The listing builds one solid part. Answer for the finished solid, in the listing's coordinates (mm). Face numbers are marked on the shaded views. A direction names the side the tool comes from. Round coordinates to 2 decimals unless told otherwise and drop trailing zeros. Loops run counter-clockwise (first coordinate to the right, second up) from the corner with the lowest first, then second, coordinate; pieces in that order, holes last. Notation, with made-up numbers: (85, 10) - (107, 10) arc R10 ccw to (107, 18) - close; hole circle Ø11 at (70, -2). An arc over 180 degrees is marked (long way). Write item = value, one per line. Start each with the question number.
1) Section B-B, the plane y = -5.3 is taken. Determine the outline of the cut face in (x, z), and give its area (3 significant figures).
2) Section C-C, the plane x = -13 is taken. Determine the outline of the cut face in (y, z).
3) Given pin 1 Ø13 at (x, z) = (5.5, 10.5) entering from +Y; pin 2 Ø3 at (x, z) = (13, 13) entering from +Y; pin 3 Ø8 at (x, z) = (-11, -11.5) entering from +Y, each flat-ended and moving along its own axis, determine where each tip first touches the part or whether it passes through.
4) Section D-D, the plane x = -4 is taken. Determine the outline of the cut face in (y, z).
5) Straight lines are drawn through the part: line 1 along Z through (x, y) = (-13, -4.3); line 2 along Z through (x, y) = (-7.5, -4.75). For each, find the intervals that lie inside material, in ascending order.
6) A tool of negligible diameter and unlimited length cuts with its end or side. For the marked faces 1, 2, 3 and 4, from which of +Z, -Z, +X, -X, +Y, -Y can it reach the whole face along a straight path? Write none if from no direction.
7) Section A-A, the plane z = 13 is taken. Determine the outline of the cut face in (x, y).
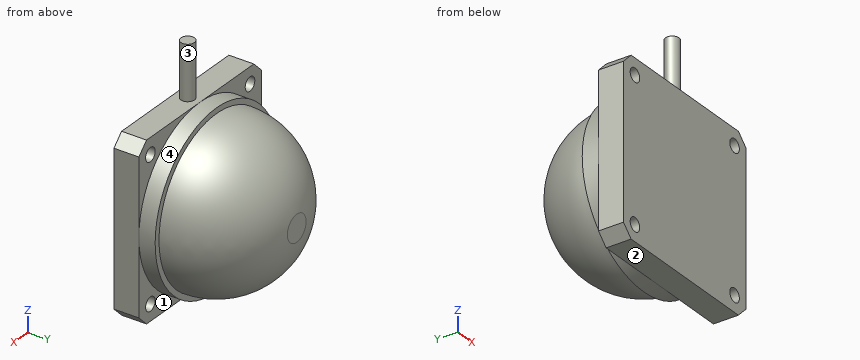
from build123d import *

# Parameters (mm, degrees)
SKETCH2_R             = 16
BOSS_EXTRUDE1_DEPTH   = 3
SKETCH3_W             = 32
SKETCH3_H             = 32
BOSS_EXTRUDE2_DEPTH   = 4.6
F_2_5MM_DOWEL_HOLE1_D = 2.5
CHAMFER1_SIZE         = 2
SKETCH11_R            = 1.25
BOSS_EXTRUDE3_DEPTH   = 10
SKETCH12_R            = 16
CUT_EXTRUDE1_DEPTH    = 38.865023439


with BuildPart() as part:
    # Sketch1 → Revolve1 (revolve)
    with BuildSketch(Plane.XY):
        with BuildLine():
            Line((0, 0), (15, 0))
            ThreePointArc((15, 0), (10.606601718, 10.606601718), (0, 15))
            Line((0, 15), (0, 0))
        make_face()
    revolve(axis=Axis((0, 15, 0), (0, -1, 0)))

    # Sketch2 → Boss-Extrude1 (add)
    with BuildSketch(Plane.XZ):
        Circle(SKETCH2_R)
    extrude(amount=BOSS_EXTRUDE1_DEPTH)

    # Sketch3 → Boss-Extrude2 (add)
    with BuildSketch(Plane.XZ.offset(3)):
        Rectangle(SKETCH3_W, SKETCH3_H)
    extrude(amount=BOSS_EXTRUDE2_DEPTH)

    # Ø2.5mm Dowel Hole1 (through all)
    with Locations(Plane(origin=(0, -3, 0), x_dir=(1, 0, 0), z_dir=(0, 1, 0))):
        with Locations((-13, 13), (13, -13), (13, 13), (-13, -13)):
            Hole(F_2_5MM_DOWEL_HOLE1_D / 2)

    # Chamfer1
    chamfer1_edges = [part.edges().sort_by_distance(p)[0] for p in [
        (16, -5.3, -16),
        (16, -5.3, 16),
        (-16, -5.3, 16),
        (-16, -5.3, -16),
    ]]
    chamfer(chamfer1_edges, length=CHAMFER1_SIZE)

    # Sketch11 → Boss-Extrude3 (add)
    with BuildSketch(Plane.XY.offset(16)):
        with Locations(Location((0, -5.3, 0), (0, 0, 180))):
            Circle(SKETCH11_R)
    extrude(amount=BOSS_EXTRUDE3_DEPTH)

    # Sketch12 → Cut-Extrude1 (cut, through all)
    with BuildSketch(Plane(origin=(0, 14.8, 0), x_dir=(1, 0, 0), z_dir=(0, 1, 0))):
        Circle(SKETCH12_R)
    extrude(amount=CUT_EXTRUDE1_DEPTH, mode=Mode.SUBTRACT)


solid = part.part
Geometry check:
q1.outline = (-16, -14) - (-14, -16) - (14, -16) - (16, -14) - (16, 14) - (14, 16) - (1.25, 16) - (1.25, 26) - (-1.25, 26) - (-1.25, 16) - (-14, 16) - (-16, 14) - close; hole circle Ø2.5 at (-13, -13); hole circle Ø2.5 at (-13, 13); hole circle Ø2.5 at (13, -13); hole circle Ø2.5 at (13, 13)
q1.area = 1,020 mm2
q2.outline = (-7.6, -16) - (-3, -16) - (-3, -14.25) - (-7.6, -14.25) - close; (-7.6, -11.75) - (-3, -11.75) - (-3, -9.33) - (0, -9.33) - (0, -7.48) arc R7.48 ccw to (0, 7.48) - (0, 9.33) - (-3, 9.33) - (-3, 11.75) - (-7.6, 11.75) - close; (-7.6, 14.25) - (-3, 14.25) - (-3, 16) - (-7.6, 16) - close
q3.pin_1 = 14.01
q3.pin_2 = -3
q3.pin_3 = 9.11
q4.outline = (-7.6, -16) - (-3, -16) - (-3, -15.49) - (0, -15.49) - (0, -14.46) arc R14.46 ccw to (0, 14.46) - (0, 15.49) - (-3, 15.49) - (-3, 16) - (-7.6, 16) - close
q5.line_1 = -16 to -14.25, -11.75 to 11.75, 14.25 to 16
q5.line_2 = -16 to 16
q6.face_1 = -Z, +X, +Y
q6.face_2 = -Z, +X, -X, +Y, -Y
q6.face_3 = +Z
q6.face_4 = +Y
q7.outline = (-16, -7.6) - (-14.25, -7.6) - (-14.25, -3) - (-16, -3) - close; (-11.75, -7.6) - (11.75, -7.6) - (11.75, -3) - (9.33, -3) - (9.33, 0) - (7.48, 0) arc R7.48 ccw to (-7.48, 0) - (-9.33, 0) - (-9.33, -3) - (-11.75, -3) - close; (14.25, -7.6) - (16, -7.6) - (16, -3) - (14.25, -3) - close
